Study the drawing (mm; zero at the part's minimum x, y, z) and answer. Coordinates: 2 decimals unless noted, no trailing zeros. Order: outer loops, then holes, each group sorted by start corner. A loop starts at its lowest first (then second) coordinate and runs counter-clockwise, first axis right, second up.
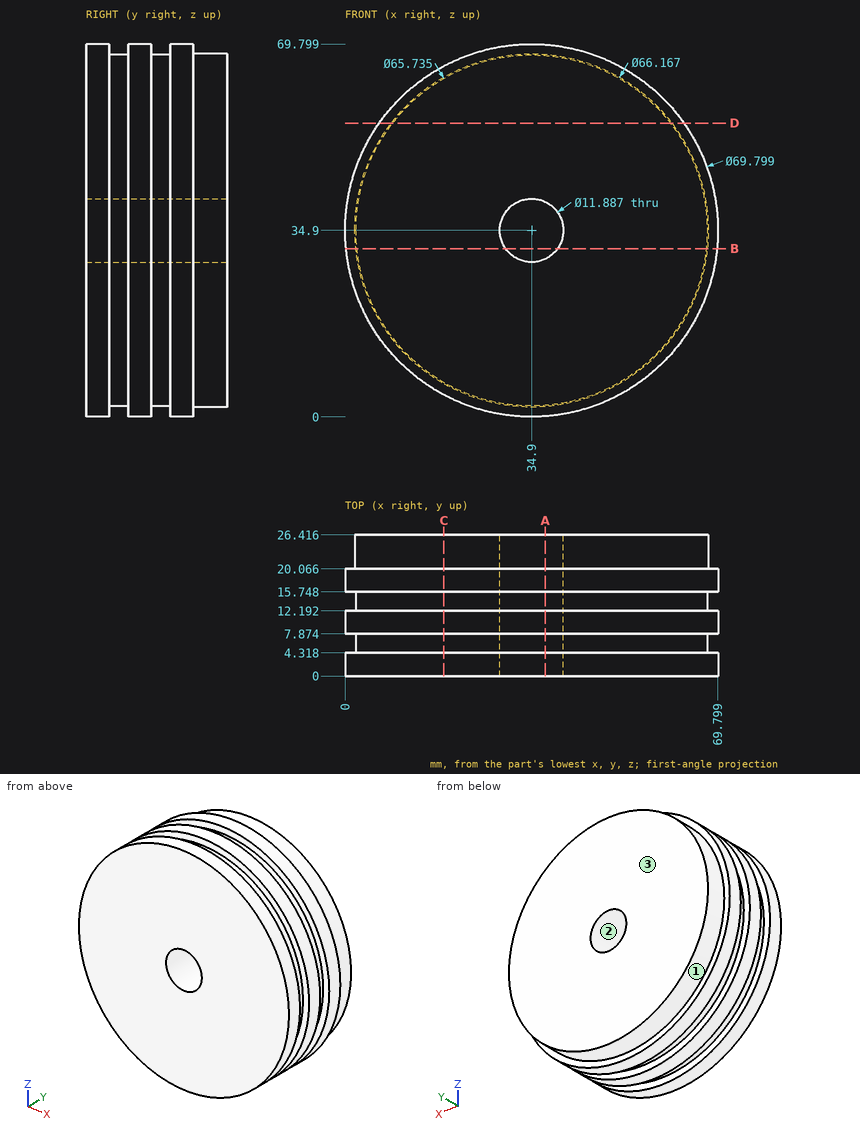
1) Straight lines are drawn through the part: line 1 (Z direction, x = 34.5, y = 13.5) (1 decimal); line 2 (X direction, y = 11.75, z = 30) (1 decimal); line 3 (Z direction, x = 32.5, y = 11.5). For each, find the intervals that lie inside material, in ascending order.
A:
line 1: z = 2 to 29, 40.8 to 67.8
line 2: x = 0.3 to 31.5, 38.3 to 69.5
line 3: z = 0.08 to 29.46, 40.34 to 69.72
2) A cutting plane is placed at A-A, the plane x = 37.5. Determine the outline of the cut face in (y, z) (1 decimal).
A:
outline: (0, 0.1) - (4.3, 0.1) - (4.3, 2.1) - (7.9, 2.1) - (7.9, 0.1) - (12.2, 0.1) - (12.2, 2.1) - (15.7, 2.1) - (15.7, 0.1) - (20.1, 0.1) - (20.1, 1.9) - (26.4, 1.9) - (26.4, 29.6) - (0, 29.6) - close; (0, 40.2) - (26.4, 40.2) - (26.4, 67.9) - (20.1, 67.9) - (20.1, 69.7) - (15.7, 69.7) - (15.7, 67.7) - (12.2, 67.7) - (12.2, 69.7) - (7.9, 69.7) - (7.9, 67.7) - (4.3, 67.7) - (4.3, 69.7) - (0, 69.7) - close
3) A cutting plane is placed at D-D, the plane z = 55. Determine the outline of the cut face in (x, y) (1 decimal).
A:
outline: (6.4, 0) - (63.4, 0) - (63.4, 4.3) - (60.9, 4.3) - (60.9, 7.9) - (63.4, 7.9) - (63.4, 12.2) - (60.9, 12.2) - (60.9, 15.7) - (63.4, 15.7) - (63.4, 20.1) - (61.2, 20.1) - (61.2, 26.4) - (8.6, 26.4) - (8.6, 20.1) - (6.4, 20.1) - (6.4, 15.7) - (8.9, 15.7) - (8.9, 12.2) - (6.4, 12.2) - (6.4, 7.9) - (8.9, 7.9) - (8.9, 4.3) - (6.4, 4.3) - close
4) Flat-ended cylindrical pins translate along their axes: pin 1 Ø12 at (y, z) = (9.5, 52) entering from -X; pin 2 Ø10 at (x, z) = (14, 8) entering from +Y; pin 3 Ø3 at (y, z) = (22.5, 26.5) entering from +X (1 decimal); pin 4 Ø3 at (x, y) = (24.5, 13) entering from -Z. Find the tip coordinate at first contact, or state that the pin passes through.
A:
pin 1: stops at x = 1.81
pin 2: stops at y = 26.42
pin 3: stops at x = 67.3
pin 4: stops at z = 1.22
5) Determine the mould class of the marked faces 1, 2 and 3 for opening direction X: pulls with the +X half, pulls with the -X half, needs draft (parallel to the pull), parting line crosses it, or undercut.
A:
face 1: parting line crosses it
face 2: undercut
face 3: needs draft
6) A cutting plane is placed at B-B, the plane z = 31.5. Determine the outline of the cut face in (x, y) (1 decimal).
A:
outline: (0.2, 0) - (30, 0) - (30, 26.4) - (2, 26.4) - (2, 20.1) - (0.2, 20.1) - (0.2, 15.7) - (2.2, 15.7) - (2.2, 12.2) - (0.2, 12.2) - (0.2, 7.9) - (2.2, 7.9) - (2.2, 4.3) - (0.2, 4.3) - close; (39.8, 0) - (69.6, 0) - (69.6, 4.3) - (67.6, 4.3) - (67.6, 7.9) - (69.6, 7.9) - (69.6, 12.2) - (67.6, 12.2) - (67.6, 15.7) - (69.6, 15.7) - (69.6, 20.1) - (67.8, 20.1) - (67.8, 26.4) - (39.8, 26.4) - close
7) A cutting plane is placed at C-C, the plane x = 18.5. Determine the outline of the cut face in (y, z) (1 decimal), and give its area (3 significant figures).
A:
outline: (0, 4.1) - (4.3, 4.1) - (4.3, 6.4) - (7.9, 6.4) - (7.9, 4.1) - (12.2, 4.1) - (12.2, 6.4) - (15.7, 6.4) - (15.7, 4.1) - (20.1, 4.1) - (20.1, 6.2) - (26.4, 6.2) - (26.4, 63.6) - (20.1, 63.6) - (20.1, 65.7) - (15.7, 65.7) - (15.7, 63.4) - (12.2, 63.4) - (12.2, 65.7) - (7.9, 65.7) - (7.9, 63.4) - (4.3, 63.4) - (4.3, 65.7) - (0, 65.7) - close
area: 1,570 mm2
